Answer from the drawing. Dimensions are ordinates in mm from the lowest x, y and z of the part. A direction names the side the tool comes from. Give positions to 0.01 mm unless a question says otherwise; leave off trailing zeros. Write each loop counter-clockwise with the first axis right and the second up, starting at its lowest first coordinate (ties: lowest second). Pieces come first, ordered by that corner, then holes. Notation, with made-up numbers: (-28.75, 49.5) -> (19.25, 49.5) arc R8 ccw to (19.25, 59.5) -> close; hole circle Ø3 at (-35, 44.25). An arc over 180 degrees is marked (long way). Write item = value, one per line.
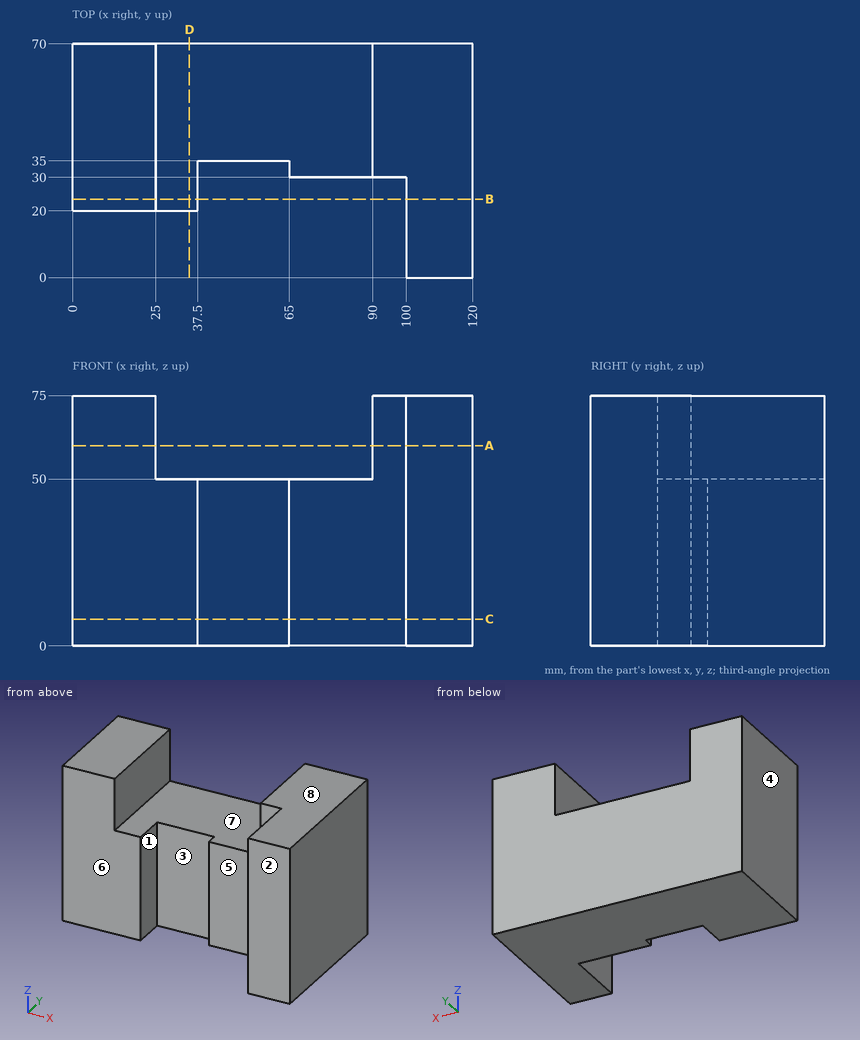
(1) Given P1, Ø2, axis at x = 12, z = 67, coming from the -Y side; P2, Ø4, axis at y = 33, z = 31, coming from the -X side; P3, Ø25, axis at x = 65.5, y = 48, coming from the +Z side; P4, Ø14, axis at x = 54, z = 21, coming from the -Y side, each flat-ended and moving along its own axis, determine where each tip first touches the part or whether it passes through.
Checks:
P1 = 20
P2 = 0
P3 = 50
P4 = 35
(2) The part is cut by section C-C on z = 8. Determine the outline of the cut face in (x, y), plus the area to 3 significant figures.
Checks:
outline = (0, 20) -> (37.5, 20) -> (37.5, 35) -> (65, 35) -> (65, 30) -> (100, 30) -> (100, 0) -> (120, 0) -> (120, 70) -> (0, 70) -> close
area = 5,640 mm²
(3) The part is cut by section B-B on y = 23.5. Determine the outline of the cut face in (x, z).
Checks:
outline = (0, 0) -> (37.5, 0) -> (37.5, 50) -> (25, 50) -> (25, 75) -> (0, 75) -> close; (100, 0) -> (120, 0) -> (120, 75) -> (100, 75) -> close
(4) For a pull along X with two mould halves and no side action, classify the marked faces 1, 2, 3 and 4 as released by +X, released by -X, zero draft, split by the parting line, or undercut.
Checks:
face_1 = undercut
face_2 = zero draft
face_3 = undercut
face_4 = released by -X
(5) A tool of negligible diameter and unlimited length cuts with its end or side. For the marked faces 5, 6, 7 and 8, from which of +Z, -Z, +X, -X, +Y, -Y can it reach the whole face along a straight path? Write none if from no direction.
Checks:
face_5 = +Z, -Z, -Y
face_6 = +Z, -Z, -X, -Y
face_7 = +Z, +Y, -Y
face_8 = +Z, +X, -X, +Y, -Y
(6) Consider L1, parallel to X at y = 55.5, z = 72.5; L2, parallel to X at y = 31, z = 5; L3, parallel to Y at x = 13, z = 44.5. Determine where each line is inside the solid, lowest interval first.
Checks:
L1 = 0 to 25, 90 to 120
L2 = 0 to 37.5, 65 to 120
L3 = 20 to 70
(7) The part is cut by section A-A on z = 60. Determine the outline of the cut face in (x, y).
Checks:
outline = (0, 20) -> (25, 20) -> (25, 70) -> (0, 70) -> close; (90, 30) -> (100, 30) -> (100, 0) -> (120, 0) -> (120, 70) -> (90, 70) -> close
(8) The part is cut by section D-D on x = 35. Determine the outline of the cut face in (y, z).
Checks:
outline = (20, 0) -> (70, 0) -> (70, 50) -> (20, 50) -> close
